```python
from build123d import *

# Parameters (mm, degrees)
BOSS_EXTRUDE2_DEPTH = 230


with BuildPart() as part:
    # Sketch1 → Boss-Extrude2 (new body)
    with BuildSketch(Plane.YZ):
        with BuildLine():
            Line((2.6, 7.124355653), (-2.6, 7.124355653))
            Line((-2.6, 7.124355653), (-2.6, 12.124355653))
            ThreePointArc((-2.6, 12.124355653), (-7.794870108, -9.643650761), (12.4, 0))
            ThreePointArc((12.4, 0), (9.643650761, 7.794870108), (2.6, 12.124355653))
            Line((2.6, 12.124355653), (2.6, 7.124355653))
        make_face()
    extrude(amount=BOSS_EXTRUDE2_DEPTH)


solid = part.part
```
Can you work these out from the model? Positions are in its coordinate system, mm. A direction names the side the tool comes from. Give positions to 0.01 mm unless a question says otherwise; leave off trailing zeros. Loops run counter-clockwise (first coordinate to the right, second up) from the corner with the lowest first, then second, coordinate; pieces in that order, holes last. Notation, with made-up numbers: M -29,88 L -10,88 A13 ccw -10,93 Z; hole C 69.25,83 d8. An arc over 180 degrees is marked long. One line per question, with ' | ' between items. Start each with the question number.
Q1. For pin 1 Ø4 at (x, y) = (89, -0.5) entering from +Z; pin 2 Ø8 at (x, y) = (175, -1.5) entering from +Z; pin 3 Ø5.5 at (x, z) = (164.5, 8.5) entering from +Y, each with a flat end and sliding along its axis, tell me the tip position at first contact or that it passes through.
Q2. For faces 3 (the flat face through (230, 0, 0)), 4 (the flat face through (113, -2.6, 10)), which set-ups out of +Z, -Z, +X, -X, +Y, -Y let a thin tool reach every point of the face, with its end or its side?
Q3. If I drill on line 1 (Y direction, x = 82, z = 0.75); line 2 (Z direction, x = 172.5, y = -1); line 3 (Y direction, x = 195.5, z = 9), over which ranges is the centre line in solid material (lowest first)? Write a range as from..to.
Q4. If we section it at A-A (x = 112.5): Please give me the cut outline in (y, z), plus the area to 3 significant figures.
Q5. If we mould it in two halves opening along Y, with no side actions, what happens to faces 1 (the flat face through (113, 0, 7.124)), 2 (the flat face through (0, 0, 0))? For each: +Y half, -Y half, draft (parallel to the pull), parting line (faces both ways), or undercut.
Q6. If we section it at B-B (y = 0): Please give me the cut outline in (x, z).
Q7. If we section it at C-C (z = -5.5): Please give me the cut outline in (x, y), plus the area to 3 significant figures.
Computed:
1) pin 1: stops at z = 7.12 | pin 2: stops at z = 12.12 | pin 3: stops at y = 10.99
2) face 3: +Z, -Z, +X, +Y, -Y | face 4: +Z, +X, -X
3) line 1: y = -12.38..12.38 | line 2: z = -12.36..7.12 | line 3: y = -8.53..-2.6, 2.6..8.53
4) outline: M -2.6,7.12 L -2.6,12.12 A12.4 ccw long 2.6,12.12 L 2.6,7.12 Z | area: 456 mm²
5) face 1: undercut | face 2: draft
6) outline: M 0,-12.4 L 230,-12.4 L 230,7.12 L 0,7.12 Z
7) outline: M 0,-11.11 L 230,-11.11 L 230,11.11 L 0,11.11 Z | area: 5,110 mm²
